```python
from build123d import *
from build123d.topology import SkipClean

# Parameters (mm, degrees)
EXTRUDE_1_DEPTH                            = 3.9
EXTRUDE_3_DEPTH                            = 20
EXTRUDE_5_DEPTH                            = 20
FILLET_1_R                                 = 0.25
FILLET_1_OF_MIRROR_2_R                     = 0.25
SKETCH_7_R                                 = 5.5
CUT_EXTRUDE_3_DEPTH                        = 69.146236458
MIRROR_3_AT_THE_SECOND_PLANE_COPY_1_SKET_R = 5.5
MIRROR_3_AT_THE_SECOND_PLANE_COPY_1_DEPTH  = 69.146236458
ESQUISSE1_W                                = 44.6
ESQUISSE1_H                                = 40
ENL_V_MAT_EXTRU_1_DEPTH                    = 1.54
ENL_V_START                                = -27.2
ENL_V_MAT_EXTRU_2_DEPTH                    = 54.4
ENL_V_MAT_EXTRU_2_2_DEPTH                  = 7.2
ENL_V_START_2                              = 20
ENL_V_MAT_EXTRU_2_3_DEPTH                  = 7.2
ESQUISSE3_W                                = 50
ESQUISSE3_H                                = 1.36
ENL_V_MAT_EXTRU_3_DEPTH                    = 64.372466761
ESQUISSE4_W                                = 27.815449133
ESQUISSE4_H                                = 40
ENL_V_MAT_EXTRU_4_DEPTH                    = 54.066651895
ESQUISSE5_R                                = 1.75
ENL_V_MAT_EXTRU_5_DEPTH                    = 54.198396436
ESQUISSE6_W                                = 13
ESQUISSE6_H                                = 18
ENL_V_MAT_EXTRU_6_DEPTH                    = 54.198396473
CONG_1_R                                   = 1
CONG_2_R                                   = 1


# Read off the part's stored shape, not the designer's step: Enl_v. mat.-Extru.2
with BuildPart() as part:
    # Sketch 1 → Extrude 1 (new body)
    with BuildSketch(Plane(origin=(0, 0, 0), x_dir=(1, 0, 0), z_dir=(0, 1, 0))):
        with BuildLine():
            Line((-40.6, -27.2), (40.6, -27.2))
            ThreePointArc((40.6, -27.2), (43.428427125, -26.028427125), (44.6, -23.2))
            Line((44.6, -23.2), (44.6, 23.2))
            ThreePointArc((44.6, 23.2), (43.428427125, 26.028427125), (40.6, 27.2))
            Line((40.6, 27.2), (-40.6, 27.2))
            ThreePointArc((-40.6, 27.2), (-43.428427125, 26.028427125), (-44.6, 23.2))
            Line((-44.6, 23.2), (-44.6, -23.2))
            ThreePointArc((-44.6, -23.2), (-43.428427125, -26.028427125), (-40.6, -27.2))
        make_face()
    extrude(amount=EXTRUDE_1_DEPTH)



with BuildPart() as body_2:
    # Sketch 3 → Extrude 3 (new, symmetric)
    with BuildSketch(Plane.XY):
        with BuildLine():
            Line((-47.815262386, -6.499919999), (-45.841869662, -6.499919999))
            ThreePointArc((-45.841869662, -6.499919999), (-44.821869662, -1.3), (-43.801869662, -6.499919999))
            Line((-43.801869662, -6.499919999), (-41.828476938, -6.499919999))
            ThreePointArc((-41.828476938, -6.499919999), (-44.821869662, -0.1), (-47.815262386, -6.499919999))
        make_face()
    extrude_3 = extrude(amount=EXTRUDE_3_DEPTH, both=True)


with BuildPart() as part_1:
    with SkipClean():  # the faces are left unmerged after this step: merging them gives an invalid solid
        add(part.part)

        add(body_2.part)  # Extrude 5 merges body 2
        # Sketch 5 → Extrude 5 (add, symmetric)
        with BuildSketch(Plane.XY):
            with BuildLine():
                Line((-36.641600827, 0.870983001), (-34.6, 0))
                ThreePointArc((-34.6, 0), (-38.684888017, -1.351535806), (-41.039960555, -4.952451312))
                Line((-41.039960555, -4.952451312), (-42.295442046, -4.952451312))
                ThreePointArc((-42.295442046, -4.952451312), (-44.821869662, -1.3), (-47.348297278, -4.952451312))
                Line((-47.348297278, -4.952451312), (-48.60377877, -4.952451312))
                ThreePointArc((-48.60377877, -4.952451312), (-44.732839073, 2.293818231), (-36.641600827, 0.870983001))
            make_face()
        extrude_5 = extrude(amount=EXTRUDE_5_DEPTH, both=True)

    # Fillet 1
    fillet_1_edges = [part_1.edges().sort_by_distance(p)[0] for p in [
        (-45.841869662, -6.499919999, 0),
        (-43.801869662, -6.499919999, 0),
    ]]
    fillet(fillet_1_edges, radius=FILLET_1_R)

    # Mirror 1: Extrude 5 across plane
    with SkipClean():  # the faces are left unmerged after this step: merging them gives an invalid solid
        add(extrude_5.mirror(Plane(origin=(0, 0, 0), x_dir=(0, 0, 1), z_dir=(1, 0, 0))))

    # Mirror 2: Extrude 3 across plane
    with SkipClean():  # the faces are left unmerged after this step: merging them gives an invalid solid
        add(extrude_3.mirror(Plane(origin=(0, 0, 0), x_dir=(0, 0, 1), z_dir=(1, 0, 0))))

    # Fillet 1 of Mirror 2
    fillet_1_of_mirror_2_edges = [part_1.edges().sort_by_distance(p)[0] for p in [
        (45.841869662, -6.499919999, 0),
        (43.801869662, -6.499919999, 0),
    ]]
    fillet(fillet_1_of_mirror_2_edges, radius=FILLET_1_OF_MIRROR_2_R)

    # Sketch 7 → Cut-Extrude 3 (cut, through all)
    with SkipClean():  # the faces are left unmerged after this step: merging them gives an invalid solid
        with BuildSketch(Plane.XY.offset(20)):
            with Locations((-45, -4)):
                Circle(SKETCH_7_R)
        cut_extrude_3 = extrude(amount=CUT_EXTRUDE_3_DEPTH, mode=Mode.SUBTRACT)

    # Mirror 3: Cut-Extrude 3 across plane
    with SkipClean():  # the faces are left unmerged after this step: merging them gives an invalid solid
        add(cut_extrude_3.mirror(Plane(origin=(0, 0, 0), x_dir=(0, 0, 1), z_dir=(1, 0, 0))), mode=Mode.SUBTRACT)

    # Mirror 3 at the second plane: Cut-Extrude 3 across plane
    with SkipClean():  # the faces are left unmerged after this step: merging them gives an invalid solid
        add(cut_extrude_3.mirror(Plane.XY), mode=Mode.SUBTRACT)

    # Mirror 3 at the second plane copy 1 sket → Mirror 3 at the second plane copy 1 (cut, through all)
    with SkipClean():  # the faces are left unmerged after this step: merging them gives an invalid solid
        with BuildSketch(Plane(origin=(0, 0, -20), x_dir=(-1, 0, 0), z_dir=(0, 0, -1))):
            with Locations((-45, -4)):
                Circle(MIRROR_3_AT_THE_SECOND_PLANE_COPY_1_SKET_R)
        extrude(amount=MIRROR_3_AT_THE_SECOND_PLANE_COPY_1_DEPTH, mode=Mode.SUBTRACT)

    # Esquisse1 → Enl_v. mat.-Extru.1 (cut)
    with SkipClean():  # the faces are left unmerged after this step: merging them gives an invalid solid
        with BuildSketch(Plane(origin=(0, 3.9, 0), x_dir=(1, 0, 0), z_dir=(0, 1, 0))):
            with Locations((-22.3, 0)):
                Rectangle(ESQUISSE1_W, ESQUISSE1_H)
        extrude(amount=-ENL_V_MAT_EXTRU_1_DEPTH, mode=Mode.SUBTRACT)

    # Enl_v. mat.-Extru.2 outline → Enl_v. mat.-Extru.2 (cut)
    with SkipClean():  # the faces are left unmerged after this step: merging them gives an invalid solid
        with BuildSketch(Plane.XY.offset(ENL_V_START)):
            with BuildLine():
                Line((0, 3.9), (0, 0))
                Line((0, 0), (34.815449133, 0))
                ThreePointArc((34.815449133, 0), (38.762946625, -1.412512906), (41.03576021, -4.935614887))
                ThreePointArc((41.03576021, -4.935614887), (41.343051607, -5.76290242), (41.828476938, -6.499919999))
                Line((41.828476938, -6.499919999), (42.913896916, -6.499919999))
                ThreePointArc((42.913896916, -6.499919999), (43.148596508, -6.33603679), (43.075589522, -6.059248812))
                ThreePointArc((43.075589522, -6.059248812), (44.821869662, -1.3), (46.568149802, -6.059248812))
                ThreePointArc((46.568149802, -6.059248812), (46.495142816, -6.33603679), (46.729842408, -6.499919999))
                Line((46.729842408, -6.499919999), (47.815262386, -6.499919999))
                ThreePointArc((47.815262386, -6.499919999), (48.623960619, -4.868391822), (48.60377877, -3.047548688))
                ThreePointArc((48.60377877, -3.047548688), (47.293490745, 0.166982283), (44.6, 2.356770326))
                Line((44.6, 2.356770326), (44.6, 3.9))
                Line((44.6, 3.9), (0, 3.9))
            make_face()
        extrude(amount=ENL_V_MAT_EXTRU_2_DEPTH, mode=Mode.SUBTRACT)

    # Enl_v. mat.-Extru.2 2 outline → Enl_v. mat.-Extru.2 2 (cut)
    with SkipClean():  # the faces are left unmerged after this step: merging them gives an invalid solid
        with BuildSketch(Plane.XY.offset(ENL_V_START)):
            with BuildLine():
                Line((0, 0), (0, 3.9))
                Line((0, 3.9), (-44.6, 3.9))
                Line((-44.6, 3.9), (-44.60000095, 1.48543533))
                ThreePointArc((-44.60000095, 1.48543533), (-42.784348631, 1.033973481), (-41.225082782, 0))
                Line((-41.225082782, 0), (0, 0))
            make_face()
        extrude(amount=ENL_V_MAT_EXTRU_2_2_DEPTH, mode=Mode.SUBTRACT)

    # Enl_v. mat.-Extru.2 3 outline → Enl_v. mat.-Extru.2 3 (cut)
    with SkipClean():  # the faces are left unmerged after this step: merging them gives an invalid solid
        with BuildSketch(Plane.XY.offset(ENL_V_START_2)):
            with BuildLine():
                Line((0, 0), (0, 3.9))
                Line((0, 3.9), (-44.6, 3.9))
                Line((-44.6, 3.9), (-44.60000095, 1.48543533))
                ThreePointArc((-44.60000095, 1.48543533), (-42.784348631, 1.033973481), (-41.225082782, 0))
                Line((-41.225082782, 0), (0, 0))
            make_face()
        extrude(amount=ENL_V_MAT_EXTRU_2_3_DEPTH, mode=Mode.SUBTRACT)

    # Esquisse3 → Enl_v. mat.-Extru.3 (cut, through all)
    with SkipClean():  # the faces are left unmerged after this step: merging them gives an invalid solid
        with BuildSketch(Plane.XY.offset(20)):
            with Locations((-25, 1.68)):
                Rectangle(ESQUISSE3_W, ESQUISSE3_H)
        extrude(amount=-ENL_V_MAT_EXTRU_3_DEPTH, mode=Mode.SUBTRACT)

    # Esquisse4 → Enl_v. mat.-Extru.4 (cut, through all)
    with SkipClean():  # the faces are left unmerged after this step: merging them gives an invalid solid
        with BuildSketch(Plane.XZ):
            with Locations((-13.907724567, 0)):
                Rectangle(ESQUISSE4_W, ESQUISSE4_H)
        extrude(amount=-ENL_V_MAT_EXTRU_4_DEPTH, mode=Mode.SUBTRACT)

    # Esquisse5 → Enl_v. mat.-Extru.5 (cut, through all)
    with SkipClean():  # the faces are left unmerged after this step: merging them gives an invalid solid
        with BuildSketch(Plane(origin=(0, 1, 0), x_dir=(1, 0, 0), z_dir=(0, 1, 0))):
            with Locations(Location((-36.905449133, 14.9, 0), (0, 0, 270))):
                Circle(ESQUISSE5_R)
            with Locations(Location((-36.905449133, -15.1, 0), (0, 0, 270))):
                Circle(ESQUISSE5_R)
        extrude(amount=-ENL_V_MAT_EXTRU_5_DEPTH, mode=Mode.SUBTRACT)

    # Esquisse6 → Enl_v. mat.-Extru.6 (cut, through all)
    with SkipClean():  # the faces are left unmerged after this step: merging them gives an invalid solid
        with BuildSketch(Plane(origin=(0, 1, 0), x_dir=(1, 0, 0), z_dir=(0, 1, 0))):
            with Locations((-34.315449133, 0)):
                Rectangle(ESQUISSE6_W, ESQUISSE6_H)
        extrude(amount=-ENL_V_MAT_EXTRU_6_DEPTH, mode=Mode.SUBTRACT)

    # Cong_1
    cong_1_edges = [part_1.edges().sort_by_distance(p)[0] for p in [
        (-40.815449133, -1.614859029, -9),
        (-40.815449133, -1.614859029, 9),
    ]]
    fillet(cong_1_edges, radius=CONG_1_R)

    # Cong_2
    cong_2_edges = [part_1.edges().sort_by_distance(p)[0] for p in [
        (-33.815449133, 1, -9),
        (-40.522555914, 1, -8.707106781),
        (-33.815449133, 1, 9),
        (-40.522555914, 1, 8.707106781),
        (-40.815449133, 1, 0),
    ]]
    fillet(cong_2_edges, radius=CONG_2_R)


solid = part_1.part
```
Design review of the part built by this model. Coordinates are the model's own, in mm. A direction names the side the tool comes from. Coordinates: 2 decimals unless noted, no trailing zeros. Order: outer loops, then holes, each group sorted by start corner. A loop starts at its lowest first (then second) coordinate and runs counter-clockwise, first axis right, second up. Notation, with made-up numbers: M 79.5,-13.5 L 136.5,-13.5 A24 ccw 136.5,23.5 Z; hole C 75.25,-23.5 d10. An arc over 180 degrees is marked long. Answer as a JSON object with one key per item and string values. Group by question number.
1) Add section A-A, the plane x = -37.75. Write out the cut boundary in (y, z).
2) Add section C-C, the plane z = -14.9. Write out the cut boundary in (x, y).
3) Tool access review of faces 4 (the flat face through (-31, 0, -15)), 5 (the flat face through (-27.815, 0.5, -14.6)), 6 (the flat face through (-44, 1, 0)), 7 (the cylindrical face through (-40.53, -1.67, 8.7)), 8 (the cylindrical face through (-33.731, 0.699, -9.285)): name each direction out of +Z, -Z, +X, -X, +Y, -Y from which nothing blocks a thin tool from reaching the whole face with its end or side.
4) Add section B-B, the plane x = -33.5. Write out the cut boundary in (y, z).
5) For pin 1 (7.5 mm diameter, centred on x = -30, z = 14.5, fed in from -Y); pin 2 (4 mm diameter, centred on x = -33, y = -3, fed in from +Z); pin 3 (5.5 mm diameter, centred on x = -36.91, z = 15.1, fed in from -Y); pin 4 (1 mm diameter, centred on y = -2.5, z = -14.5, fed in from +X), all flat-tipped, find the tip position at first contact; note any pin that passes through.
6) Add section D-D, the plane z = -4. Write out the cut boundary in (x, y), then the cut area to 3 significant figures.
7) Mouldability with a two-part tool opening along Z and no side actions: class faces 1 (the flat face through (-41, -1, 20)), 2 (the flat face through (-41, -1, -20)), 3 (the flat face through (-39, -1, -9)) as pulls with the +Z half, pulls with the -Z half, needs draft (parallel to the pull), parting line crosses it, or undercut.
8) Wall thickness on L1, parallel to X at y = -4, z = -5.5; L2, parallel to Z at x = -39.5, y = -0.5; L3, parallel to Y at x = -29.25, z = -12.5: over which ranges is each line inside the solid? List them lowest first.
Computed values:
{
 "1": {"outline": "M -0.75,-20 L 1,-20 L 1,-16.43 L -0.75,-16.43 Z; M -0.75,-13.37 L 1,-13.37 L 1,-10 A1 ccw 0,-9 L -0.75,-9 Z; M -0.75,9 L 0,9 A1 ccw 1,10 L 1,13.57 L -0.75,13.57 Z; M -0.75,16.63 L 1,16.63 L 1,20 L -0.75,20 Z"},
 "2": {"outline": "M -48.6,-3.05 A3.9 ccw -47.82,-6.5 L -46.73,-6.5 A0.25 ccw -46.57,-6.06 A2.7 cw long -43.08,-6.06 A0.25 ccw -42.91,-6.5 L -41.83,-6.5 A3.9 ccw -41.04,-4.94 A6.52 cw -38.66,-1.33 L -38.66,1 L -46.57,1 A7 ccw Z; M -35.16,-0.01 A6.52 cw -34.82,0 L -27.82,0 L -27.82,1 L -35.16,1 Z"},
 "3": {"face 4": "+Z, -Z, +X, -Y", "face 5": "+Z, -Z, +X, +Y, -Y", "face 6": "+Z, -Z, +X, -X, +Y", "face 7": "+X, +Y, -Y", "face 8": "+X, +Y"},
 "4": {"outline": "M 0,-20 L 1,-20 L 1,-10 A1 ccw 0,-9 Z; M 0,9 A1 ccw 1,10 L 1,20 L 0,20 Z"},
 "5": {"pin 1": "stops at y = 0", "pin 2": "passes through", "pin 3": "stops at y = -2.28", "pin 4": "stops at x = -39.41"},
 "6": {"outline": "M -48.6,-3.05 A3.9 ccw -47.82,-6.5 L -46.73,-6.5 A0.25 ccw -46.57,-6.06 A2.7 cw long -43.08,-6.06 A0.25 ccw -42.91,-6.5 L -41.83,-6.5 A3.9 ccw -41.04,-4.94 A6.52 cw -40.82,-4.23 L -40.82,0 A1 ccw -41.82,1 L -46.57,1 A7 ccw Z", "area": "31.1 mm^2"},
 "7": {"face 1": "pulls with the +Z half", "face 2": "pulls with the -Z half", "face 3": "undercut"},
 "8": {"L1": "x = -48.72 to -47.52, -42.12 to -40.82", "L2": "z = -20 to -9, 9 to 20", "L3": "y = 0 to 1"}
}
